Check sheet for the modelled part. Datum: model origin and axes. Units: mm. Round coordinates to 2 decimals unless told otherwise and drop trailing zeros. Loops run counter-clockwise (first coordinate to the right, second up) from the corner with the lowest first, then second, coordinate; pieces in that order, holes last. Notation, with made-up numbers: (-1, 59) - (7, 59) arc R29 cw to (7, 93) - close; hole circle Ø3 at (77.5, -19.75). An arc over 180 degrees is marked (long way). Put each result on its own line as item: value. Start each with the question number.
Item 1: Section check B-B, the plane x = 39.5. Record the cut outline in (y, z), and give its area (3 significant figures).
Item 2: Draft check along X on faces 1 (the cylindrical face through (-60.47, -46.367, 187.34)), 2 (the cylindrical face through (74.74, 23.54, 187.34)), 3 (the flat face through (17, -75, 0)). Enter one of: pulls with the +X half, pulls with the -X half, needs draft (parallel to the pull), parting line crosses it, or undercut.
Item 3: Section check A-A, the plane y = 0. Record the cut outline in (x, z).
Item 4: Material ranges on line 1 along Y through (x, z) = (0, 216.5); line 2 along Y through (x, z) = (-2, 358); line 3 along X through (y, z) = (-42.5, 76.5), recorded low to high.
Item 5: Gauge pin test, flat ends, axial feed: pin 1 Ø1.5 at (x, z) = (-30.5, 95.5) entering from +Y; pin 2 Ø6 at (y, z) = (51.5, 243) entering from +X; pin 3 Ø5 at (y, z) = (12, 44) entering from -X. Record the tip position at first contact, or that the pin passes through.
Item 6: Section check C-C, the plane z = 200. Record the cut outline in (x, y), and give its area (3 significant figures).
from build123d import *

# Parameters (mm, degrees)
SKETCH1_R           = 78.359
SKETCH1_R_2         = 76.2
BOSS_EXTRUDE1_DEPTH = 380
SKETCH5_W           = 2.25
SKETCH5_H           = 78.359
CIRPATTERN2_COUNT   = 6


with BuildPart() as part:
    # Sketch1 → Boss-Extrude1 (new body)
    with BuildSketch(Plane.XY):
        Circle(SKETCH1_R)
        Circle(SKETCH1_R_2, mode=Mode.SUBTRACT)
    extrude(amount=BOSS_EXTRUDE1_DEPTH)

    # Sketch5 → M4 Clearance Hole2 (revolve, cut)
    with BuildSketch(Plane(origin=(0, 0, 10), x_dir=(0, 0, -1), z_dir=(1, 0, 0))):
        with Locations((1.125, 39.1795)):
            Rectangle(SKETCH5_W, SKETCH5_H)
    m4_clearance_hole2 = revolve(axis=Axis((0, -6.35, 10), (0, 1, 0)), mode=Mode.SUBTRACT)

    # CirPattern2: M4 Clearance Hole2 ×6 about axis
    cirpattern2_axis = Axis((0, 0, 380), (0, 0, -1))
    for i in range(1, CIRPATTERN2_COUNT):
        add(m4_clearance_hole2.rotate(cirpattern2_axis, i * 360 / CIRPATTERN2_COUNT), mode=Mode.SUBTRACT)


solid = part.part
Check result:
1. outline: (-67.67, 0) - (-65.16, 0) - (-65.16, 380) - (-67.67, 380) - close; (65.16, 0) - (67.67, 0) - (67.67, 380) - (65.16, 380) - close
1. area: 1,910 mm²
2. face 1: undercut
2. face 2: parting line crosses it
2. face 3: needs draft
3. outline: (-78.36, 0) - (-76.2, 0) - (-76.2, 380) - (-78.36, 380) - close; (76.2, 0) - (78.36, 0) - (78.36, 380) - (76.2, 380) - close
4. line 1: -78.36 to -76.2, 76.2 to 78.36
4. line 2: -78.33 to -76.17, 76.17 to 78.33
4. line 3: -65.83 to -63.25, 63.25 to 65.83
5. pin 1: y = 72.49
5. pin 2: x = 61.55
5. pin 3: x = -77.78
6. outline: circle Ø156.72 at (0, 0); hole circle Ø152.4 at (0, 0)
6. area: 1,050 mm²
